Could you check a few things on this model? Use its own coordinates, in mm. Face numbers are marked on the shaded views. A direction names the side the tool comes from. Round coordinates to 2 decimals unless told otherwise and drop trailing zeros. Order: outer loops, then holes, each group sorted by start corner. A loop starts at its lowest first (then second) coordinate and runs counter-clockwise, first axis right, second up. Notation, with made-up numbers: (27.25, 1) - (69.25, 1) arc R22 ccw to (69.25, 30) - close; hole circle Ø2 at (81.25, 72). An arc over 180 degrees is marked (long way). Return JSON: item names as keys, results as strings. Group by question number.
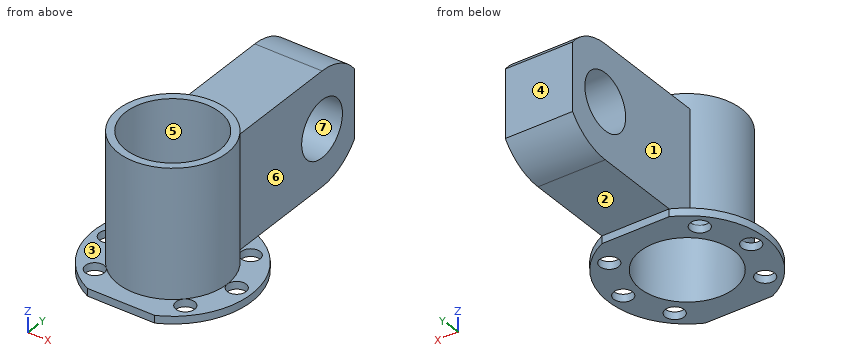
from build123d import *

# Parameters (mm, degrees)
IZIM1_R                          = 14.5
IZIM1_R_2                        = 12.5
Y_KSEKLIK_EKSTR_ZYON1_DEPTH      = 34
IZIM2_R                          = 21
IZIM2_R_2                        = 12.5
Y_KSEKLIK_EKSTR_ZYON2_DEPTH      = 2
IZIM3_R                          = 2.5
KES_EKSTR_ZYON1_DEPTH            = 78
KES_EKSTR_ZYON2_DEPTH            = 78
Y_KSEKLIK_EKSTR_ZYON5_REACH      = 54.146
Y_KSEKLIK_EKSTR_ZYON5_END_RADIUS = 14.5
IZIM6_W                          = 30
IZIM6_H                          = 17.88854382
Y_KSEKLIK_EKSTR_ZYON6_DEPTH      = 40
IZIM10_R                         = 7.5
KES_EKSTR_ZYON3_DEPTH            = 30
KES_EKSTR_ZYON4_DEPTH            = 93


with BuildPart() as part:
    # izim1 → Y_kseklik-Ekstr_zyon1 (new body)
    with BuildSketch(Plane.XY):
        Circle(IZIM1_R)
        Circle(IZIM1_R_2, mode=Mode.SUBTRACT)
    extrude(amount=Y_KSEKLIK_EKSTR_ZYON1_DEPTH)



with BuildPart() as body_2:
    # izim2 → Y_kseklik-Ekstr_zyon2 (new body)
    with BuildSketch(Plane(origin=(0, 0, 0), x_dir=(-1, 0, 0), z_dir=(0, 0, -1))):
        Circle(IZIM2_R)
        with Locations(Location((0, 0, 0), (0, 0, 180))):
            Circle(IZIM2_R_2, mode=Mode.SUBTRACT)
    extrude(amount=Y_KSEKLIK_EKSTR_ZYON2_DEPTH)

    # izim3 → Kes-Ekstr_zyon1 (cut)
    with BuildSketch(Plane(origin=(0, 0, -2), x_dir=(-1, 0, 0), z_dir=(0, 0, -1))):
        with Locations((-17, 0)):
            Circle(IZIM3_R)
        with Locations((-12.02081528, 12.02081528)):
            Circle(IZIM3_R)
        with Locations((12.02081528, 12.02081528)):
            Circle(IZIM3_R)
        with Locations((17, 0)):
            Circle(IZIM3_R)
        with Locations((12.02081528, -12.02081528)):
            Circle(IZIM3_R)
        with Locations((-12.02081528, -12.02081528)):
            Circle(IZIM3_R)
    extrude(amount=-KES_EKSTR_ZYON1_DEPTH, mode=Mode.SUBTRACT)

    # izim4 → Kes-Ekstr_zyon2 (cut)
    with BuildSketch(Plane(origin=(0, 0, -2), x_dir=(-1, 0, 0), z_dir=(0, 0, -1))):
        with BuildLine():
            Line((-8.94427191, 19), (8.94427191, 19))
            ThreePointArc((8.94427191, 19), (0, 21), (-8.94427191, 19))
        make_face()
        with BuildLine():
            Line((-8.94427191, -19), (8.94427191, -19))
            ThreePointArc((8.94427191, -19), (0, -21), (-8.94427191, -19))
        make_face()
    extrude(amount=-KES_EKSTR_ZYON2_DEPTH, mode=Mode.SUBTRACT)


with BuildPart() as part_1:
    add(part.part)

    add(body_2.part)  # Y_kseklik-Ekstr_zyon5 merges body 2
    # Y_kseklik-Ekstr_zyon5: up to this cylinder (the profile starts outside it)
    y_kseklik_ekstr_zyon5_end = Plane(origin=(0, 0, 15), z_dir=(0, 0, -1)) * Cylinder(Y_KSEKLIK_EKSTR_ZYON5_END_RADIUS, 138.292, mode=Mode.PRIVATE)
    # izim6 → Y_kseklik-Ekstr_zyon5 (add, up to the surface)
    with BuildSketch(Plane(origin=(0, 14.5, 0), x_dir=(0, 0, -1), z_dir=(0, 1, 0)), mode=Mode.PRIVATE) as y_kseklik_ekstr_zyon5_sk1:
        with Locations((-15, 0)):
            Rectangle(IZIM6_W, IZIM6_H)
    y_kseklik_ekstr_zyon5_tool1 = extrude(y_kseklik_ekstr_zyon5_sk1.sketch, amount=-Y_KSEKLIK_EKSTR_ZYON5_REACH, mode=Mode.PRIVATE) - y_kseklik_ekstr_zyon5_end
    add(y_kseklik_ekstr_zyon5_tool1.solids().sort_by_distance((0, 14.5, 15))[0])
    add(y_kseklik_ekstr_zyon5_tool1.solids().sort_by_distance((0, 14.5, 15))[1])

    # izim9 → Y_kseklik-Ekstr_zyon6 (add)
    with BuildSketch(Plane(origin=(0, 14.5, 0), x_dir=(1, 0, 0), z_dir=(0, 1, 0))):
        Polygon((-8.94427191, -30), (0, -30), (8.94427191, -30), (8.94427191, 0), (-8.94427191, 0), align=None)
    extrude(amount=Y_KSEKLIK_EKSTR_ZYON6_DEPTH)

    # izim10 → Kes-Ekstr_zyon3 (cut)
    with BuildSketch(Plane.ZY.offset(8.94427191)):
        with Locations(Location((15, 42.5, 0), (0, 0, 270))):
            Circle(IZIM10_R)
    extrude(amount=-KES_EKSTR_ZYON3_DEPTH, mode=Mode.SUBTRACT)

    # izim11 → Kes-Ekstr_zyon4 (cut)
    with BuildSketch(Plane.ZY.offset(8.94427191)):
        with BuildLine():
            Line((30, 42.5), (30, 54.5))
            Line((30, 54.5), (24, 54.5))
            ThreePointArc((24, 54.5), (28.416407865, 49.208203932), (30, 42.5))
        make_face()
        with BuildLine():
            Line((0, 54.5), (6, 54.5))
            ThreePointArc((6, 54.5), (1.583592135, 49.208203932), (0, 42.5))
            Line((0, 42.5), (0, 54.5))
        make_face()
    extrude(amount=-KES_EKSTR_ZYON4_DEPTH, mode=Mode.SUBTRACT)


solid = part_1.part
1) I want a section at B-B, the plane y = 41.5. List the corners of the cut face in (x, z) for me, plus the area to 3 significant figures.
2) For the marked faces 1, 2, 3 and 4, which set-ups out of +Z, -Z, +X, -X, +Y, -Y let a thin tool reach every point of the face, with its end or its side?
3) I want a section at C-C, the plane z = 3. List the corners of the cut face in (x, y) for me, plus the area to 3 significant figures.
4) If I drill on line 1 along Y through (x, z) = (-8, 19); line 2 along Y through (x, z) = (-6, 20.5); line 3 along X through (y, z) = (22.5, 19), over which ranges is the centre line in solid material (lowest first)? Write a range as from..to.
5) I want a section at A-A, the plane x = 0. List the corners of the cut face in (y, z) for me.
6) We'd pull the mould along X, two halves only. Please class the marked faces 5, 6 and 7: +X half, -X half, draft (parallel to the pull), parting line (faces both ways), or undercut.
7) I want a section at D-D, the plane x = -17. List the corners of the cut face in (y, z) for me, plus the area to 3 significant figures.
8) Will these pins go through, and if not, where does the flat tip stop? pin 1 (10 mm diameter, centred on x = 4, y = 40, fed in from +Z); pin 2 (9 mm diameter, centred on y = 24, z = 15, fed in from -X); pin 3 (1 mm diameter, centred on x = -5.5, z = 8.5, fed in from -Y); pin 4 (4 mm diameter, centred on x = -17, y = 0, fed in from +Z).
Outcome:
{
 "1": {"outline": "(-8.94, 0) - (8.94, 0) - (8.94, 7.57) - (-8.94, 7.57) - close; (-8.94, 22.43) - (8.94, 22.43) - (8.94, 30) - (-8.94, 30) - close", "area": "271 mm^2"},
 "2": {"face 1": "+Z, -X, +Y", "face 2": "-Z, +X, -X, +Y", "face 3": "+Z", "face 4": "+Z, -Z, +X, -X, +Y"},
 "3": {"outline": "(-8.94, 11.41) arc R14.5 ccw (long way) to (8.94, 11.41) - (8.94, 51.5) - (-8.94, 51.5) - close; hole circle Ø25 at (0, 0)", "area": "849 mm^2"},
 "4": {"line 1": "-12.09..-9.6, 9.6..36.16, 48.84..54.5", "line 2": "-13.2..-10.97, 10.97..37.4, 47.6..54.5", "line 3": "-8.94..8.94"},
 "5": {"outline": "(-19, -2) - (-12.5, -2) - (-12.5, 34) - (-14.5, 34) - (-14.5, 0) - (-19, 0) - close; (12.5, -2) - (19, -2) - (19, 0) - (42.5, 0) arc R15 ccw to (54.5, 6) - (54.5, 24) arc R15 ccw to (42.5, 30) - (14.5, 30) - (14.5, 34) - (12.5, 34) - close; hole circle Ø15 at (42.5, 15)"},
 "6": {"face 5": "undercut", "face 6": "+X half", "face 7": "draft"},
 "7": {"outline": "(-12.33, -2) - (-2.5, -2) - (-2.5, 0) - (-12.33, 0) - close; (2.5, -2) - (12.33, -2) - (12.33, 0) - (2.5, 0) - close", "area": "39.3 mm^2"},
 "8": {"pin 1": "z = 30", "pin 2": "x = -8.94", "pin 3": "y = -13.61", "pin 4": "through"}
}
